Source: three-view drawing plus pictorial views. Frame: mm from the lowest corner of the part. A direction names the side the tool comes from. Round coordinates to 2 decimals unless told otherwise and drop trailing zeros. Loops run counter-clockwise (first coordinate to the right, second up) from the corner with the lowest first, then second, coordinate; pieces in that order, holes last. Notation, with made-up numbers: (-12.5, -23) -> (41.5, -23) arc R28 cw to (41.5, 2) -> close; hole circle Ø10 at (-35, 54.25). An arc over 180 degrees is marked (long way). Answer in a Markdown table with one row per item.
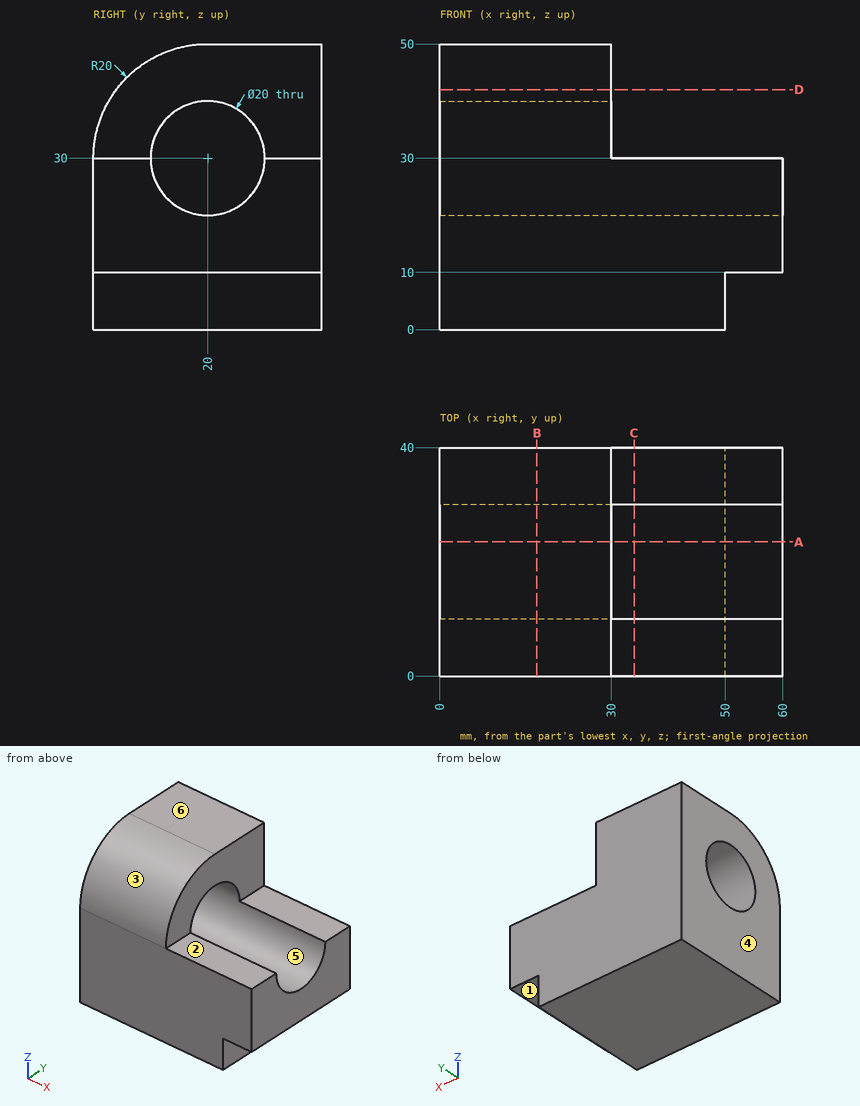
Item 1: Cut plane A-A (y = 23.5). Output: boundary loops of the cut face in (x, z), then the cut area to 3 significant figures.
Answer:
| item | result |
|---|---|
| outline | (0, 0) -> (50, 0) -> (50, 10) -> (60, 10) -> (60, 20.63) -> (0, 20.63) -> close; (0, 39.37) -> (30, 39.37) -> (30, 50) -> (0, 50) -> close |
| area | 1,460 mm² |
Item 2: Cut plane C-C (x = 34). Output: boundary loops of the cut face in (y, z), then the cut area to 3 significant figures.
Answer:
| item | result |
|---|---|
| outline | (0, 0) -> (40, 0) -> (40, 30) -> (30, 30) arc R10 cw to (10, 30) -> (0, 30) -> close |
| area | 1,040 mm² |
Item 3: Line query: probe 1 along Y at (x, z) = (13, 29.5); probe 2 along Z at (x, y) = (21.5, 20); probe 3 along X at (y, z) = (33, 46). Output: solid intervals per line, ascending. Write a range as [from, to].
Answer:
| item | result |
|---|---|
| probe 1 | y = [0, 10.01], [29.99, 40] |
| probe 2 | z = [0, 20], [40, 50] |
| probe 3 | x = [0, 30] |
Item 4: Pin query (flat end, axial travel): pin 1 Ø8 at (y, z) = (30, 7) entering from +X; pin 2 Ø11 at (x, y) = (51.5, 6.5) entering from +Z; pin 3 Ø5 at (x, y) = (56.5, 23) entering from -Z; pin 4 Ø6 at (y, z) = (24, 40) entering from +X. Return the tip coordinate at first contact, or that it passes through.
Answer:
| item | result |
|---|---|
| pin 1 | stops at x = 60 |
| pin 2 | stops at z = 30 |
| pin 3 | stops at z = 10 |
| pin 4 | stops at x = 30 |
Item 5: Cut plane D-D (z = 42). Output: boundary loops of the cut face in (x, y), then the cut area to 3 significant figures.
Answer:
| item | result |
|---|---|
| outline | (0, 4) -> (30, 4) -> (30, 40) -> (0, 40) -> close |
| area | 1,080 mm² |
Item 6: Cut plane B-B (x = 17). Output: boundary loops of the cut face in (y, z), then the cut area to 3 significant figures.
Answer:
| item | result |
|---|---|
| outline | (0, 0) -> (40, 0) -> (40, 50) -> (20, 50) arc R20 ccw to (0, 30) -> close; hole circle Ø20 at (20, 30) |
| area | 1,600 mm² |
Item 7: Reachability of the marked faces 1, 2 and 3 from +Z, -Z, +X, -X, +Y, -Y: full face, straight path, thin tool, end or side. Return the list, or none.
Answer:
| item | result |
|---|---|
| face 1 | -Z, +X, +Y, -Y |
| face 2 | +Z, +X, +Y, -Y |
| face 3 | +Z, +X, -X, -Y |
Item 8: Draft query along Z for the marked faces 4, 5 and 6. Return one class per face: pulls with the +Z half, pulls with the -Z half, needs draft (parallel to the pull), parting line crosses it, or undercut.
Answer:
| item | result |
|---|---|
| face 4 | needs draft |
| face 5 | undercut |
| face 6 | pulls with the +Z half |
